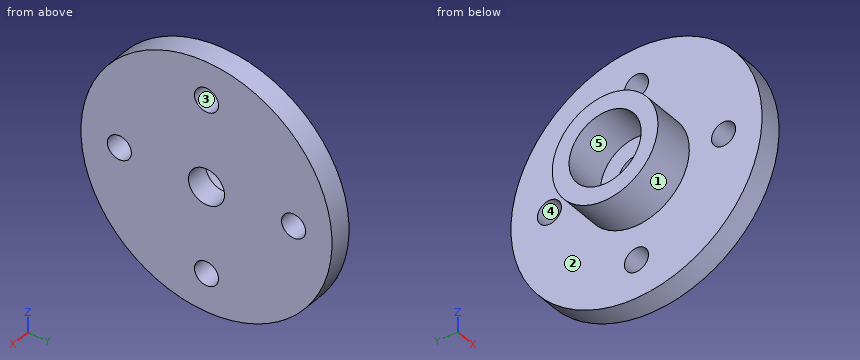
from build123d import *

# Parameters (mm, degrees)
SKETCH1_R           = 4.4
SKETCH1_R_2         = 3
BOSS_EXTRUDE1_DEPTH = 3.5
SKETCH2_R           = 10.45
BOSS_EXTRUDE2_DEPTH = 1.9
SKETCH3_R           = 1.5
CUT_EXTRUDE1_DEPTH  = 1.9
SKETCH4_R           = 1
CUT_EXTRUDE2_DEPTH  = 5.4


with BuildPart() as part:
    # Sketch1 → Boss-Extrude1 (new body)
    with BuildSketch(Plane(origin=(0, 0, 0), x_dir=(0, 0, -1), z_dir=(1, 0, 0))):
        Circle(SKETCH1_R)
        Circle(SKETCH1_R_2, mode=Mode.SUBTRACT)
    extrude(amount=BOSS_EXTRUDE1_DEPTH)

    # Sketch2 → Boss-Extrude2 (add)
    with BuildSketch(Plane(origin=(3.5, 0, 0), x_dir=(0, 0, -1), z_dir=(1, 0, 0))):
        with Locations(Location((0, 0, 0), (0, 0, 180))):
            Circle(SKETCH2_R)
    extrude(amount=BOSS_EXTRUDE2_DEPTH)

    # Sketch3 → Cut-Extrude1 (cut)
    with BuildSketch(Plane(origin=(5.4, 0, 0), x_dir=(0, 0, -1), z_dir=(1, 0, 0))):
        Circle(SKETCH3_R)
    extrude(amount=-CUT_EXTRUDE1_DEPTH, mode=Mode.SUBTRACT)

    # Sketch4 → Cut-Extrude2 (cut)
    with BuildSketch(Plane(origin=(5.4, 0, 0), x_dir=(0, 0, -1), z_dir=(1, 0, 0))):
        with Locations((0, 7.25)):
            Circle(SKETCH4_R)
        with Locations((7.25, 0)):
            Circle(SKETCH4_R)
        with Locations((0, -7.25)):
            Circle(SKETCH4_R)
        with Locations((-7.25, 0)):
            Circle(SKETCH4_R)
    extrude(amount=-CUT_EXTRUDE2_DEPTH, mode=Mode.SUBTRACT)


solid = part.part
Verification items for the finished model (mm, model axes). Face numbers are marked on the shaded views. A direction names the side the tool comes from. Give positions to 0.01 mm unless a question says otherwise; leave off trailing zeros. Loops run counter-clockwise (first coordinate to the right, second up) from the corner with the lowest first, then second, coordinate; pieces in that order, holes last. Notation, with made-up numbers: (-32.75, 17.5) - (14.25, 17.5) arc R32 cw to (14.25, 51.5) - close; hole circle Ø3 at (79.25, 57.25). An arc over 180 degrees is marked (long way). Write item = value, one per line. Start each with the question number.
Q1. Cross-section at B-B, the plane z = 7.25. Enter the section's corners in (x, y).
Q2. Tool access check on the marked faces 4 and 5. Record the directions out of +Z, -Z, +X, -X, +Y, -Y that give a thin tool (end or side, any length) a straight path to the whole face; none if there is none.
Q3. Cross-section at C-C, the plane y = -6.75. Enter the section's corners in (x, z), and give its area (3 significant figures).
Q4. Thickness scan on line 1 (Y direction, x = 3.9, z = 0); line 2 (Y direction, x = 2.35, z = 0); line 3 (X direction, y = -4.75, z = 7). Record the ranges inside material, lowest first.
Q5. Depth check by flat-ended pin: P1, Ø1.8, axis at y = 0, z = -7.25, coming from the -X side; P2, Ø2.5, axis at y = -7.25, z = 0, coming from the +X side; P3, Ø3, axis at x = 3.5, y = -7.5, coming from the +Z side; P4, Ø2, axis at x = 4, z = -5, coming from the +Y side. Enter the tip coordinate at first touch or a pass-through.
Q6. Cross-section at A-A, the plane z = 0. Enter the section's corners in (x, y), and give its area (3 significant figures).
Q7. Cross-section at D-D, the plane x = 1.2. Enter the section's corners in (y, z), and give its area (3 significant figures).
Q8. Mould release check, pull along Y, two halves, no side actions. Record for the marked faces 1, 2 and 3: released by +Y, released by -Y, zero draft, split by the parting line, or undercut.
Answer key:
q1.outline = (3.5, -7.53) - (5.4, -7.53) - (5.4, -1) - (3.5, -1) - close; (3.5, 1) - (5.4, 1) - (5.4, 7.53) - (3.5, 7.53) - close
q2.face_4 = +X, -X
q2.face_5 = -X
q3.outline = (3.5, -7.98) - (5.4, -7.98) - (5.4, -0.87) - (3.5, -0.87) - close; (3.5, 0.87) - (5.4, 0.87) - (5.4, 7.98) - (3.5, 7.98) - close
q3.area = 27.0 mm^2
q4.line_1 = -10.45 to -8.25, -6.25 to -1.5, 1.5 to 6.25, 8.25 to 10.45
q4.line_2 = -4.4 to -3, 3 to 4.4
q4.line_3 = 3.5 to 5.4
q5.P1 = through
q5.P2 = 5.4
q5.P3 = 8.56
q5.P4 = 9.65
q6.outline = (0, -4.4) - (3.5, -4.4) - (3.5, -6.25) - (5.4, -6.25) - (5.4, -1.5) - (3.5, -1.5) - (3.5, -3) - (0, -3) - close; (0, 3) - (3.5, 3) - (3.5, 1.5) - (5.4, 1.5) - (5.4, 6.25) - (3.5, 6.25) - (3.5, 4.4) - (0, 4.4) - close; (3.5, -10.45) - (5.4, -10.45) - (5.4, -8.25) - (3.5, -8.25) - close; (3.5, 8.25) - (5.4, 8.25) - (5.4, 10.45) - (3.5, 10.45) - close
q6.area = 36.2 mm^2
q7.outline = circle Ø8.8 at (0, 0); hole circle Ø6 at (0, 0)
q7.area = 32.5 mm^2
q8.face_1 = split by the parting line
q8.face_2 = zero draft
q8.face_3 = undercut
